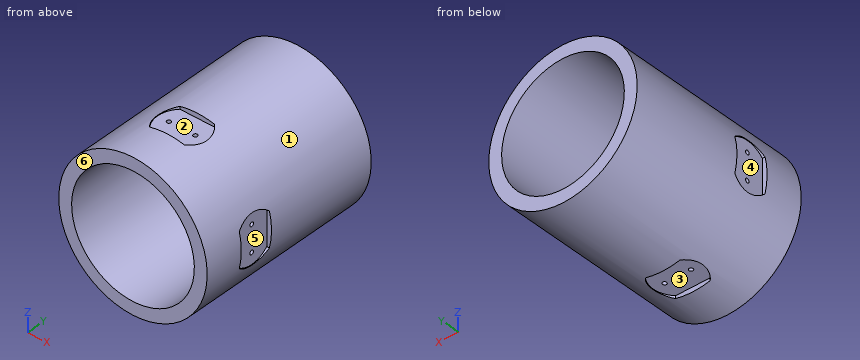
from build123d import *

# Parameters (mm, degrees)
SKETCH2_R           = 39.3
SKETCH2_R_2         = 32.5
BOSS_EXTRUDE1_DEPTH = 100
CUT_EXTRUDE1_START  = 39.3
CUT_EXTRUDE1_DEPTH  = 2.5
SKETCH4_R           = 1.1
CUT_EXTRUDE2_DEPTH  = 3
CIRPATTERN1_COUNT   = 4


with BuildPart() as part:
    # Sketch2 → Boss-Extrude1 (new body)
    with BuildSketch(Plane(origin=(0, 0, 0), x_dir=(1, 0, 0), z_dir=(0, 1, 0))):
        with Locations(Location((0, 0, 0), (0, 0, 270))):
            Circle(SKETCH2_R)
        with Locations(Location((0, 0, 0), (0, 0, 270))):
            Circle(SKETCH2_R_2, mode=Mode.SUBTRACT)
    extrude(amount=BOSS_EXTRUDE1_DEPTH)

    # Sketch3 → Cut-Extrude1 (cut)
    with BuildSketch(Plane.XY.offset(CUT_EXTRUDE1_START)):
        with BuildLine():
            Line((9.192388155, 39.192388155), (-9.192388155, 39.192388155))
            ThreePointArc((-9.192388155, 39.192388155), (-13, 30), (-9.192388155, 20.807611845))
            Line((-9.192388155, 20.807611845), (9.192388155, 20.807611845))
            ThreePointArc((9.192388155, 20.807611845), (13, 30), (9.192388155, 39.192388155))
        make_face()
    cut_extrude1 = extrude(amount=-CUT_EXTRUDE1_DEPTH, mode=Mode.SUBTRACT)

    # Sketch4 → Cut-Extrude2 (cut)
    with BuildSketch(Plane.XY.offset(36.8)):
        with Locations((7, 30)):
            Circle(SKETCH4_R)
        with Locations((-7, 30)):
            Circle(SKETCH4_R)
    cut_extrude2 = extrude(amount=-CUT_EXTRUDE2_DEPTH, mode=Mode.SUBTRACT)

    # CirPattern1: Cut-Extrude1, Cut-Extrude2 ×4 about axis
    cirpattern1_axis = Axis((0, 0, 0), (0, 1, 0))
    add([cut_extrude1.rotate(cirpattern1_axis, i * 360 / CIRPATTERN1_COUNT) for i in range(1, CIRPATTERN1_COUNT)], mode=Mode.SUBTRACT)
    add([cut_extrude2.rotate(cirpattern1_axis, i * 360 / CIRPATTERN1_COUNT) for i in range(1, CIRPATTERN1_COUNT)], mode=Mode.SUBTRACT)


solid = part.part
Build history of the part. All positions in model axes, mm. Face numbers are marked on the shaded views. A direction names the side the tool comes from. Round coordinates to 2 decimals unless told otherwise and drop trailing zeros. Write each loop counter-clockwise with the first axis right and the second up, starting at its lowest first coordinate (ties: lowest second). Pieces come first, ordered by that corner, then holes. Notation, with made-up numbers: M -22.5,59.25 L -16.5,59.25 A19 cw -16.5,86.25 Z; hole C -29,-32.5 d2. An arc over 180 degrees is marked long. Answer in a Markdown table with one row per item.
1. Saw through at D-D (x = -24). List the corners of the cut face in (y, z).
Geometry check:
| item | result |
|---|---|
| outline | M 0,-31.12 L 100,-31.12 L 100,-21.91 L 0,-21.91 Z; M 0,21.91 L 100,21.91 L 100,31.12 L 0,31.12 Z |
2. Saw through at B-B (x = 0). List the corners of the cut face in (y, z), and give its area (3 significant figures).
Geometry check:
| item | result |
|---|---|
| outline | M 0,-39.3 L 20.81,-39.3 L 20.81,-36.8 L 39.19,-36.8 L 39.19,-39.3 L 100,-39.3 L 100,-32.5 L 0,-32.5 Z; M 0,32.5 L 100,32.5 L 100,39.3 L 39.19,39.3 L 39.19,36.8 L 20.81,36.8 L 20.81,39.3 L 0,39.3 Z |
| area | 1,270 mm2 |
3. Mould opens along Z. For the marked faces 1, 2, 3 and 4 say: +Z half, -Z half, draft (parallel to the pull), parting line (faces both ways), or undercut.
Geometry check:
| item | result |
|---|---|
| face 1 | parting line |
| face 2 | +Z half |
| face 3 | -Z half |
| face 4 | undercut |
4. Flat gauge pins, fed straight in: P1, Ø5.5, axis at y = 30, z = -3, coming from the -X side; P2, Ø1.3, axis at y = 30, z = 7, coming from the +X side; P3, Ø1.5, axis at y = 87, z = -7.5, coming from the +X side. Where does each tip first touch, or does it go through?
Geometry check:
| item | result |
|---|---|
| P1 | x = -36.8 |
| P2 | x = 33.8 |
| P3 | x = 38.72 |
5. Saw through at C-C (y = 27). List the corners of the cut face in (x, z), and give its area (3 significant figures).
Geometry check:
| item | result |
|---|---|
| outline | M -37.21,-12.65 A39.3 ccw -12.65,-37.21 L -12.65,-36.8 L 12.65,-36.8 L 12.65,-37.21 A39.3 ccw 37.21,-12.65 L 36.8,-12.65 L 36.8,12.65 L 37.21,12.65 A39.3 ccw 12.65,37.21 L 12.65,36.8 L -12.65,36.8 L -12.65,37.21 A39.3 ccw -37.21,12.65 L -36.8,12.65 L -36.8,-12.65 Z; hole C 0,0 d65 |
| area | 1,350 mm2 |
6. Which spindle directions (+Z, -Z, +X, -X, +Y, -Y) get a long thin tool onto all of the face, cutting with end or side? Do the marked faces 5 and 6. Say none if no direction does.
Geometry check:
| item | result |
|---|---|
| face 5 | +X |
| face 6 | +Z, -Z, +X, -X, -Y |
7. Probe L1, parallel to X at y = 30, z = 0; L2, parallel to X at y = 58.5, z = 0; L3, parallel to Y at x = 7, z = 36. List the from-to ranges inside material, lowest first. Write a range as [from, to].
Geometry check:
| item | result |
|---|---|
| L1 | [-36.8, -32.5], [32.5, 36.8] |
| L2 | [-39.3, -32.5], [32.5, 39.3] |
| L3 | [0, 28.9], [31.1, 100] |
8. Saw through at A-A (z = 0). List the corners of the cut face in (x, y).
Geometry check:
| item | result |
|---|---|
| outline | M -39.3,0 L -32.5,0 L -32.5,100 L -39.3,100 L -39.3,39.19 L -36.8,39.19 L -36.8,20.81 L -39.3,20.81 Z; M 32.5,0 L 39.3,0 L 39.3,20.81 L 36.8,20.81 L 36.8,39.19 L 39.3,39.19 L 39.3,100 L 32.5,100 Z |
